Autodesk Inventor part; units mm, degrees
ref_plane "YZ Plane" through (0, 0, 0) normal (1, 0, 0) x (0, 1, 0)
ref_plane "XZ Plane" through (0, 0, 0) normal (0, 1, 0) x (-1, 0, 0)
ref_plane "XY Plane" through (0, 0, 0) normal (0, 0, 1) x (1, 0, 0)
sketch "Boceto1" plane through (0, 0, 0) normal (0, 0, 1) x (1, 0, 0)
  line L0 (0, 1.5671) -> (-5, 1.5671)
  line L1 (-5, 1.5671) -> (-5, 1.2168)
  line L2 (-1.5, 1.1) -> (-5, 1.2168)
  line L3 (-1.5, 1.1) -> (-1.5, 0.8)
  line L4 (-1.5, 0.8) -> (-0.75, 0.8)
  line L5 (-0.75, 0.8) -> (-0.75, 0)
  line L6 (-0.75, 0) -> (0, 0)
  line L7 (0, 0) -> (0, 1.5671)
revolve "Revolución1" add sketch "Boceto1" angle 360 about axis through (0, 0, 0) along (0, 1, 0)
sketch "Boceto2" plane through (0, 1.5671, 0) normal (0, 1, 0) x (1, 0, 0)
  line L0 (0, 0) -> (-0.75, 0)
  circle A0 centre (0, 0) radius 0.75
  line L1 (-0.75, 0) -> (-0.75, 0.75)
  line L2 (-0.75, 0.75) -> (0.75, 0.75)
  line L3 (0.75, 0.75) -> (0.75, -0.75)
  line L4 (0.75, -0.75) -> (-0.75, -0.75)
  line L5 (-0.75, -0.75) -> (-0.75, 0)
  dimension "d1" = 0.75
  dimension "d2" = 0.75
  dimension "d3" = 1.5
  dimension "d4" = 1.5
  dimension "d5" = 1.5
extrude "Extrusión1" add sketch "Boceto2" along normal blind 0.8
properties part number "enlacecuello"
Work out the finished part from the listing and answer in its coordinate system (mm). A direction names the side the tool comes from. Round coordinates to 2 decimals unless told otherwise and drop trailing zeros. Loops run counter-clockwise (first coordinate to the right, second up) from the corner with the lowest first, then second, coordinate; pieces in that order, holes last. Notation, with made-up numbers: (9, 32.5) -> (38, 32.5) arc R18 cw to (38, 47.5) -> close; hole circle Ø6 at (-15.75, 45.25). An arc over 180 degrees is marked (long way). Write each question's results on one line, items separated by ' | '. Start each with the question number.
1. Find the intervals of material crossed by probe 1 along Y at (x, z) = (1, 2.75); probe 2 along Y at (x, z) = (-2, 3.25); probe 3 along X at (y, z) = (1.45, 4), in increasing order. Write a range as from..to.
2. Section C-C (y = 0.45) is taken. Determine the outline of the cut face in (x, z).
3. For a pull along Z with two mould halves and no side action, classify faces 5 (the face through (0, 2, 0.75)), 6 (the face through (0, 2, -0.75)), 7 (the face through (0, 0, 0)) as +Z half, -Z half, draft (parallel to the pull), parting line (faces both ways), or undercut.
4. Section B-B (x = 0) is taken. Determine the outline of the cut face in (y, z), plus the area to 3 significant figures.
5. Section A-A (z = 0) is taken. Determine the outline of the cut face in (x, y), plus the area to 3 significant figures.
6. A tool of negligible diameter and unlimited length cuts with its end or side. For faces 1 (the face through (0, 2.367, 0)), 2 (the face through (1.5, 0.95, -0.07)), 3 (the face through (-0.75, 2, 0)), 4 (the face through (0.75, 2, 0)), from which of +Z, -Z, +X, -X, +Y, -Y can it reach the whole face along a straight path? Write none if from no direction.
7. Section D-D (y = 2.2) is taken. Determine the outline of the cut face in (x, z).
8. Given pin 1 Ø1 at (x, y) = (3, 1.5) entering from +Z; pin 2 Ø0.6 at (y, z) = (2, 0) entering from +X; pin 3 Ø0.6 at (x, y) = (0, 2) entering from +Z, each flat-ended and moving along its own axis, determine where each tip first touches the part or whether it passes through.
Evaluation:
1) probe 1: y = 1.15..1.57 | probe 2: y = 1.18..1.57 | probe 3: x = -3..3
2) outline: circle Ø1.5 at (0, 0)
3) face 5: +Z half | face 6: -Z half | face 7: draft
4) outline: (0, -0.75) -> (0.8, -0.75) -> (0.8, -1.5) -> (1.1, -1.5) -> (1.22, -5) -> (1.57, -5) -> (1.57, -0.75) -> (2.37, -0.75) -> (2.37, 0.75) -> (1.57, 0.75) -> (1.57, 5) -> (1.22, 5) -> (1.1, 1.5) -> (0.8, 1.5) -> (0.8, 0.75) -> (0, 0.75) -> close | area: 7.56 mm2
5) outline: (-5, 1.22) -> (-1.5, 1.1) -> (-1.5, 0.8) -> (-0.75, 0.8) -> (-0.75, 0) -> (0.75, 0) -> (0.75, 0.8) -> (1.5, 0.8) -> (1.5, 1.1) -> (5, 1.22) -> (5, 1.57) -> (0.75, 1.57) -> (0.75, 2.37) -> (-0.75, 2.37) -> (-0.75, 1.57) -> (-5, 1.57) -> close | area: 7.56 mm2
6) face 1: +Z, -Z, +X, -X, +Y | face 2: -Y | face 3: +Z, -Z, -X, +Y | face 4: +Z, -Z, +X, +Y
7) outline: (-0.75, -0.75) -> (0.75, -0.75) -> (0.75, 0.75) -> (-0.75, 0.75) -> close
8) pin 1: stops at z = 4.33 | pin 2: stops at x = 0.75 | pin 3: stops at z = 0.75
